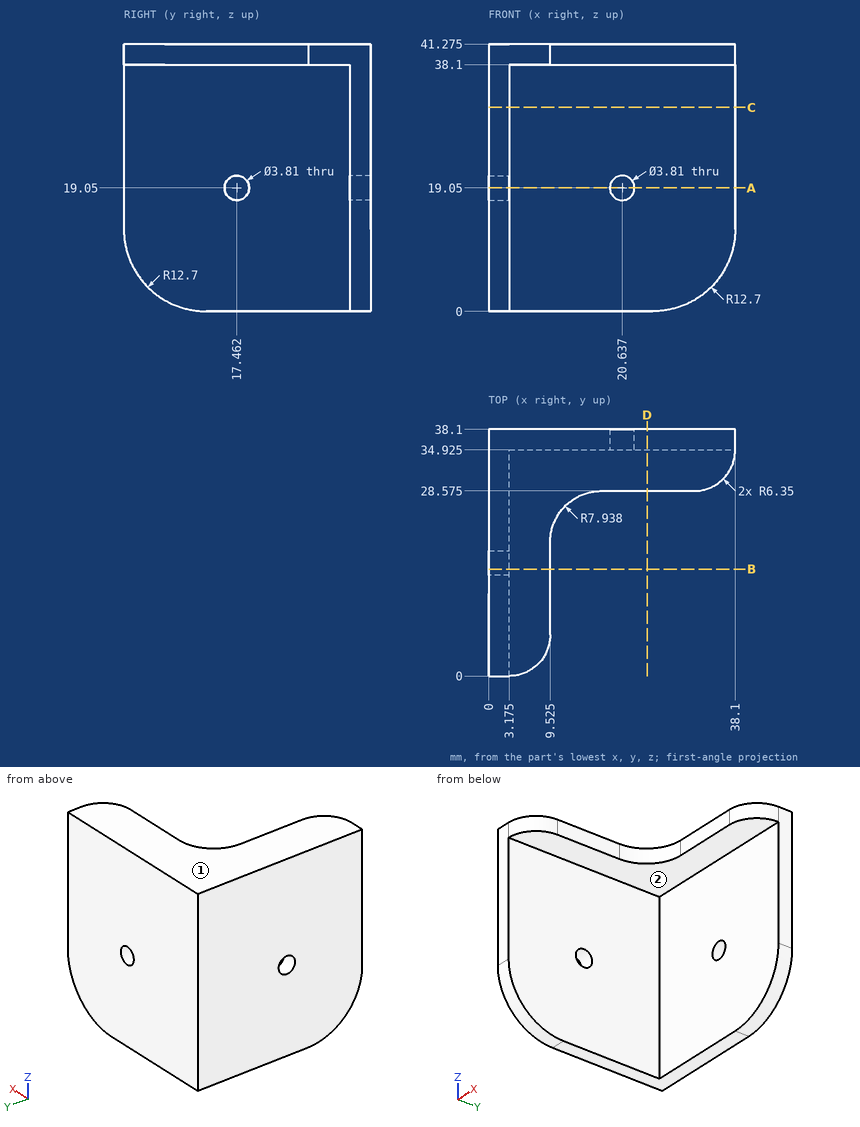
Verification items for this drawing (mm, ordinates from the low corner). A direction names the side the tool comes from. Coordinates: 2 decimals unless noted, no trailing zeros. Write each loop counter-clockwise with the first axis right and the second up, starting at its lowest first coordinate (ties: lowest second). Pieces come first, ordered by that corner, then holes. Notation, with made-up numbers: M 46.5,54.5 L 55.5,54.5 A15 ccw 55.5,76.5 Z; hole C 13,49.5 d5. An arc over 180 degrees is marked long. Use CSV: the item, a comma, the result in double quotes.
Q1. Set-up check for the marked faces 1 and 2: record each of +Z, -Z, +X, -X, +Y, -Y from which the full face is reachable in a straight line by a thin tool's end or side.
Computed values:
face 1,"+Z, +X, -X, +Y, -Y"
face 2,"-Z, +X, -Y"
Q2. Section check B-B, the plane y = 16.5. Enter the section's corners in (x, z) (1 decimal), and give its area (3 significant figures).
Computed values:
outline,"M 0,0 L 3.2,0 L 3.2,17.4 L 0,17.4 Z; M 0,20.7 L 3.2,20.7 L 3.2,38.1 L 9.5,38.1 L 9.5,41.3 L 0,41.3 Z"
area,"141 mm²"
Q3. Section check D-D, the plane x = 24.5. Enter the section's corners in (y, z) (1 decimal), and give its area (3 significant figures).
Computed values:
outline,"M 28.6,38.1 L 34.9,38.1 L 34.9,0 L 38.1,0 L 38.1,41.3 L 28.6,41.3 Z"
area,"151 mm²"
Q4. Thickness scan on line 1 along Y through (x, z) = (1, 19); line 2 along X through (y, z) = (35, 19); line 3 along Y through (x, z) = (5.5, 30.5) (1 decimal). Record the ranges inside material, lowest first. Write a range as [from, to].
Computed values:
line 1,"[0, 15.56], [19.37, 38.1]"
line 2,"[0, 18.73], [22.54, 38.1]"
line 3,"[34.9, 38.1]"
Q5. Section check A-A, the plane z = 19.05. Enter the section's corners in (x, y) (1 decimal).
Computed values:
outline,"M 0,0 L 3.2,0 L 3.2,15.6 L 0,15.6 Z; M 0,19.4 L 3.2,19.4 L 3.2,34.9 L 18.7,34.9 L 18.7,38.1 L 0,38.1 Z; M 22.5,34.9 L 38.1,34.9 L 38.1,38.1 L 22.5,38.1 Z"
Q6. Section check C-C, the plane z = 31.5. Enter the section's corners in (x, y) (1 decimal), and give its area (3 significant figures).
Computed values:
outline,"M 0,0 L 3.2,0 L 3.2,34.9 L 38.1,34.9 L 38.1,38.1 L 0,38.1 Z"
area,"232 mm²"
Q7. Go/stop test with flat-tipped pins: P1, Ø10.5, axis at x = 24.5, y = 23, coming from the -Z side; P2, Ø8, axis at x = 10.5, z = 11.5, coming from the -Y side (1 decimal); P3, Ø1, axis at x = 25, z = 40, coming from the -Y side (1 decimal); P4, Ø1, axis at y = 10.5, z = 39, coming from the +X side (1 decimal). Record where each tip stops, or that it passes through.
Computed values:
P1,"through"
P2,"y = 34.9"
P3,"y = 28.6"
P4,"x = 9.5"
